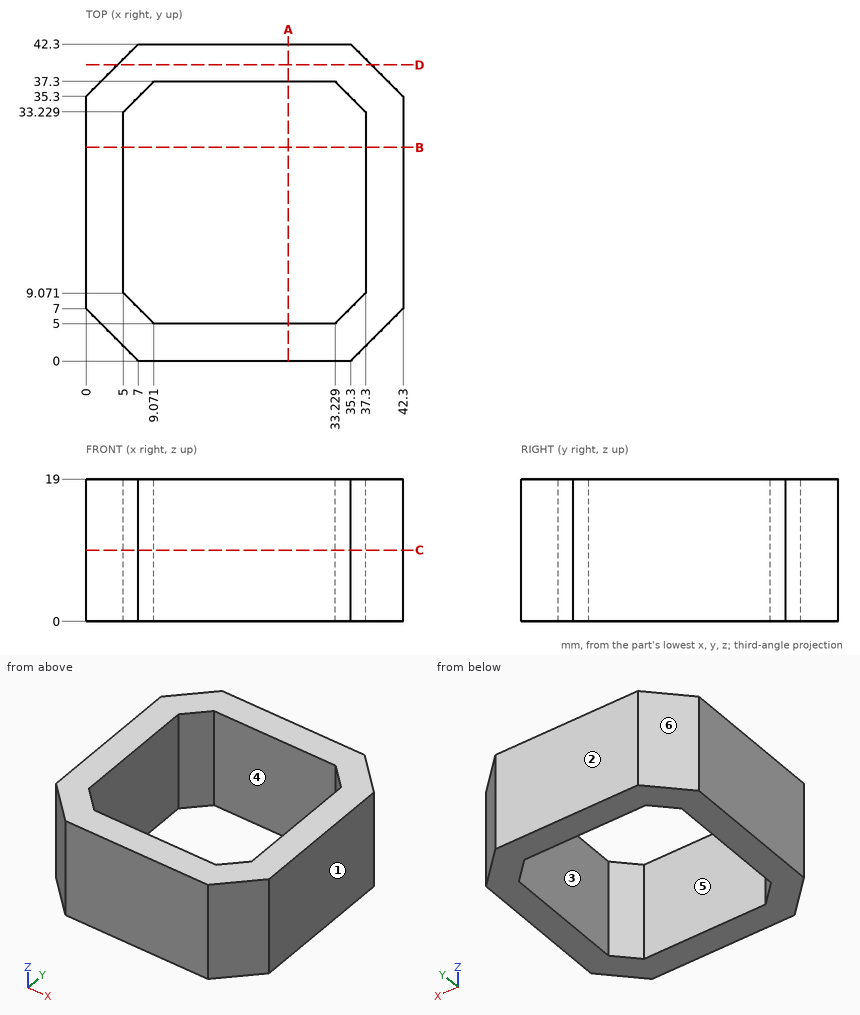
Answer from the drawing. Dimensions are ordinates in mm from the lowest x, y and z of the part. A direction names the side the tool comes from. Coordinates: 2 decimals unless noted, no trailing zeros. Write each loop counter-clockwise with the first axis right and the second up, starting at its lowest first coordinate (ties: lowest second). Pieces come first, ordered by that corner, then holes. Notation, with made-up numbers: M 85,-6 L 113,-6 A12 cw 113,12 Z; hole C 26.5,-7.75 d4. An arc over 180 degrees is marked long. Put each result on its own line as item: value. Start each with the question number.
1. For a pull along Y with two mould halves and no side action, classify the marked faces 1, 2, 3 and 4 as pulls with the +Y half, pulls with the -Y half, needs draft (parallel to the pull), parting line crosses it, or undercut.
2. A cutting plane is placed at A-A on x = 27. Write down the section's boundary in (y, z).
3. A cutting plane is placed at D-D on y = 39.5. Write down the section's boundary in (x, z), then the cut area to 3 significant figures.
4. Which of the six approach directions +Z, -Z, +X, -X, +Y, -Y give full straight-line access (tool end or side, diameter ignored) to the marked faces 5 and 6?
5. A cutting plane is placed at C-C on z = 9.5. Write down the section's boundary in (x, y), then the cut area to 3 significant figures.
6. Consider line 1 (Y direction, x = 23.5, z = 1.25); line 2 (X direction, y = 9, z = 11.25). Determine where each line is inside the solid, lowest interval first. Write a range as from..to.
7. A flat-ended cylindrical pin translates along its axis: P1, Ø9.5, axis at y = 25.5, z = 9.5, coming from the -X side. Find the tip coordinate at first contact, or state that the pin passes through.
Resolved:
1. face 1: needs draft
1. face 2: pulls with the +Y half
1. face 3: undercut
1. face 4: undercut
2. outline: M 0,0 L 5,0 L 5,19 L 0,19 Z; M 37.3,0 L 42.3,0 L 42.3,19 L 37.3,19 Z
3. outline: M 4.2,0 L 38.1,0 L 38.1,19 L 4.2,19 Z
3. area: 644 mm2
4. face 5: +Z, -Z
4. face 6: +Z, -Z, -X, +Y
5. outline: M 0,7 L 7,0 L 35.3,0 L 42.3,7 L 42.3,35.3 L 35.3,42.3 L 7,42.3 L 0,35.3 Z; hole M 5,9.07 L 9.07,5 L 33.23,5 L 37.3,9.07 L 37.3,33.23 L 33.23,37.3 L 9.07,37.3 L 5,33.23 Z
5. area: 681 mm2
6. line 1: y = 0..5, 37.3..42.3
6. line 2: x = 0..5.07, 37.23..42.3
7. P1: stops at x = 0
